Geometry: final body of the model. Coordinates: model frame, mm. A direction names the side the tool comes from. Give positions to 0.01 mm unless a question says otherwise; leave off trailing zeros. Write each loop counter-clockwise with the first axis right and the second up, starting at its lowest first coordinate (ties: lowest second). Pieces come first, ordered by that corner, then holes.
from build123d import *

# Parameters (mm, degrees)
F0_W     = 45.5000007218
F0_H     = 20.0000007218
F0_W_2   = 42.5
F0_H_2   = 17
F0_R     = 1.7580829865
F1_DEPTH = 1.5
F2_DEPTH = 14
F3_W     = 17
F3_H     = 13.5
F4_DEPTH = 2


with BuildPart() as f1:
    # F0 (on Top) → F1 (new body)
    with BuildSketch(Plane.XY):
        with Locations((1.4756151661, 0.1818094146)):
            Rectangle(F0_W, F0_H)
        with Locations((1.4756151661, 0.1818094146)):
            Rectangle(F0_W_2, F0_H_2, mode=Mode.SUBTRACT)
        with Locations((1.4756151661, 0.1818094146)):
            Rectangle(F0_W_2, F0_H_2)
        with Locations((18.9648512751, -4.5714476146)):
            Circle(F0_R, mode=Mode.SUBTRACT)
    extrude(amount=-F1_DEPTH)

    # F0 (on Top) → F2 (join)
    with BuildSketch(Plane.XY):
        with Locations((1.4756151661, 0.1818094146)):
            Rectangle(F0_W, F0_H)
        with Locations((1.4756151661, 0.1818094146)):
            Rectangle(F0_W_2, F0_H_2, mode=Mode.SUBTRACT)
    extrude(amount=F2_DEPTH)

    # F3 (on face) → F4 (cut)
    with BuildSketch(Plane.XZ.offset(9.8181909463)):
        with Locations((11.725615527, 6.75)):
            Rectangle(F3_W, F3_H)
    extrude(amount=-F4_DEPTH, mode=Mode.SUBTRACT)


solid = f1.part
Q1. Pull-direction query (Z, two-part tool) for faces 1 (the flat face through (1, 10.182, 6)), 2 (the flat face through (12, -9, 13.5)), 3 (the flat face through (1, 0, -1.5)); classes: released by +Z, released by -Z, zero draft, split by the parting line, or undercut.
Filled sheet:
face 1: zero draft
face 2: undercut
face 3: released by -Z
Q2. Section A-A on x = 7. Output: boundary loops of the cut face in (y, z).
Filled sheet:
outline: (-9.82, -1.5) - (10.18, -1.5) - (10.18, 14) - (8.68, 14) - (8.68, 0) - (-9.82, 0) - close; (-9.82, 13.5) - (-8.32, 13.5) - (-8.32, 14) - (-9.82, 14) - close
Q3. Ray query, line 1 along X through (y, z) = (7.5, 11); line 2 along Y through (x, z) = (-10.5, 3); line 3 along Z through (x, y) = (13, -8.5). Return the intervals inside material, ascending.
Filled sheet:
line 1: x = -21.27 to -19.77, 22.73 to 24.23
line 2: y = -9.82 to -8.32, 8.68 to 10.18
line 3: z = -1.5 to 0, 13.5 to 14
Q4. Pin query (flat end, axial travel): P1, Ø4.5, axis at x = 18.96, y = -4.57, coming from the +Z side. Return the tip coordinate at first contact, or that it passes through.
Filled sheet:
P1: stops at z = 0
Q5. Section D-D on x = 19. Output: boundary loops of the cut face in (y, z), plus the area to 3 significant figures.
Filled sheet:
outline: (-9.82, -1.5) - (-6.33, -1.5) - (-6.33, 0) - (-9.82, 0) - close; (-9.82, 13.5) - (-8.32, 13.5) - (-8.32, 14) - (-9.82, 14) - close; (-2.81, -1.5) - (10.18, -1.5) - (10.18, 14) - (8.68, 14) - (8.68, 0) - (-2.81, 0) - close
area: 46.5 mm2
Q6. Section C-C on z = 2. Output: boundary loops of the cut face in (x, y).
Filled sheet:
outline: (-21.27, -9.82) - (3.23, -9.82) - (3.23, -8.32) - (-19.77, -8.32) - (-19.77, 8.68) - (22.73, 8.68) - (22.73, -8.32) - (20.23, -8.32) - (20.23, -9.82) - (24.23, -9.82) - (24.23, 10.18) - (-21.27, 10.18) - close
Q7. Section B-B on y = -7.5. Output: boundary loops of the cut face in (x, z), plus the area to 3 significant figures.
Filled sheet:
outline: (-21.27, -1.5) - (24.23, -1.5) - (24.23, 14) - (22.73, 14) - (22.73, 0) - (-19.77, 0) - (-19.77, 14) - (-21.27, 14) - close
area: 110 mm2
Q8. Access query for faces 4 (the cylindrical face through (17.21, -4.49, -0.74)), 5 (the flat face through (22.726, 0, 7)), 6 (the flat face through (3.226, -9, 7)). Directions: +Z, -Z, +X, -X, +Y, -Y. A direction counts if a zero-diameter tool reaches every point of the face in a straight line with its end or side. Return the directions, or none.
Filled sheet:
face 4: +Z, -Z
face 5: +Z
face 6: -Y
